Here's the drawing with two shaded views (mm, measured from the low corner). I have some questions. A direction names the side the tool comes from. Round coordinates to 2 decimals unless told otherwise and drop trailing zeros. Loops run counter-clockwise (first coordinate to the right, second up) from the corner with the lowest first, then second, coordinate; pieces in that order, holes last. Notation, with made-up numbers: (18, -6) - (35, -6) arc R7 ccw to (35, 2) - close; hole circle Ø10 at (-19.75, 30.25). An arc over 180 degrees is marked (long way). Use one line per item in the form item = value.
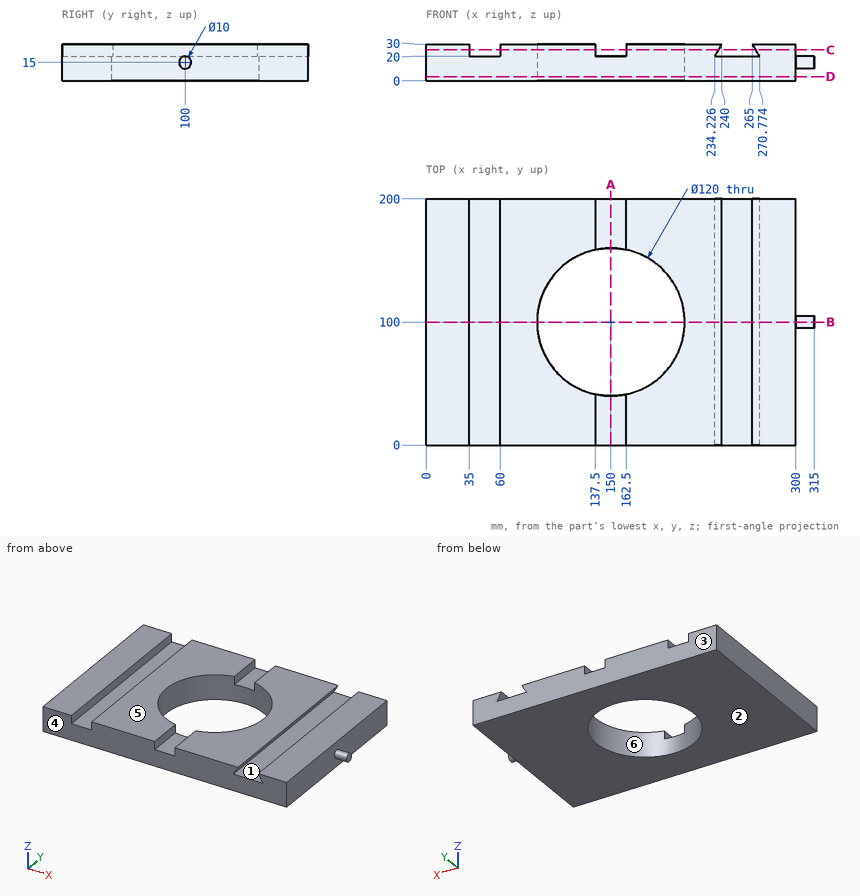
1. If we section it at A-A, the plane x = 150: Write out the boundary of the cut face in (y, z).
Solution:
outline = (0, 0) - (40, 0) - (40, 20) - (0, 20) - close; (160, 0) - (200, 0) - (200, 20) - (160, 20) - close
2. For P1, Ø11, axis at y = 23.5, z = 23.5, coming from the -X side; P2, Ø12.5, axis at x = 154.5, y = 28, coming from the +Z side; P3, Ø10, axis at y = 132, z = 11.5, coming from the +X side; P4, Ø5, axis at x = 94.5, y = 98, coming from the -Z side, each with a flat end and sliding along its axis, tell me the tip position at first contact or that it passes through.
Solution:
P1 = 0
P2 = 20
P3 = 300
P4 = through
3. If we section it at B-B, the plane y = 100: Write out the boundary of the cut face in (x, z), plus the area to 3 significant figures.
Solution:
outline = (0, 0) - (90, 0) - (90, 30) - (60, 30) - (60, 20) - (35, 20) - (35, 30) - (0, 30) - close; (210, 0) - (300, 0) - (300, 10) - (315, 10) - (315, 20) - (300, 20) - (300, 30) - (265, 30) - (270.77, 20) - (234.23, 20) - (240, 30) - (210, 30) - close
area = 4,990 mm^2
4. We'd pull the mould along Y, two halves only. Please class the marked faces 3, 4, 5 and 6: +Y half, -Y half, draft (parallel to the pull), parting line (faces both ways), or undercut.
Solution:
face_3 = +Y half
face_4 = -Y half
face_5 = draft
face_6 = undercut
5. If we section it at C-C, the plane z = 25.25: Write out the boundary of the cut face in (x, y).
Solution:
outline = (0, 0) - (35, 0) - (35, 200) - (0, 200) - close; (60, 0) - (137.5, 0) - (137.5, 41.32) arc R60 cw to (137.5, 158.68) - (137.5, 200) - (60, 200) - close; (162.5, 0) - (237.26, 0) - (237.26, 200) - (162.5, 200) - (162.5, 158.68) arc R60 cw to (162.5, 41.32) - close; (267.74, 0) - (300, 0) - (300, 200) - (267.74, 200) - close
6. On a 3-axis mill with a long thin cutter (end or side, diameter ignored), from which of +Z, -Z, +X, -X, +Y, -Y can I reach the whole of each face in a straight line? I mean the marked faces 1 and 2. Say none if no direction works.
Solution:
face_1 = +Y, -Y
face_2 = -Z, +X, -X, +Y, -Y
7. If we section it at D-D, the plane z = 3.5: Write out the boundary of the cut face in (x, y).
Solution:
outline = (0, 0) - (300, 0) - (300, 200) - (0, 200) - close; hole circle Ø120 at (150, 100)
8. Please list where these lines run through material, in increasing order: line 1 along X through (y, z) = (100, 8.75); line 2 along Y through (x, z) = (150, 15.5); line 3 along X through (y, z) = (51.5, 24.75) (1 decimal).
Solution:
line_1 = 0 to 90, 210 to 300
line_2 = 0 to 40, 160 to 200
line_3 = 0 to 35, 60 to 114.7, 185.3 to 237, 268 to 300
